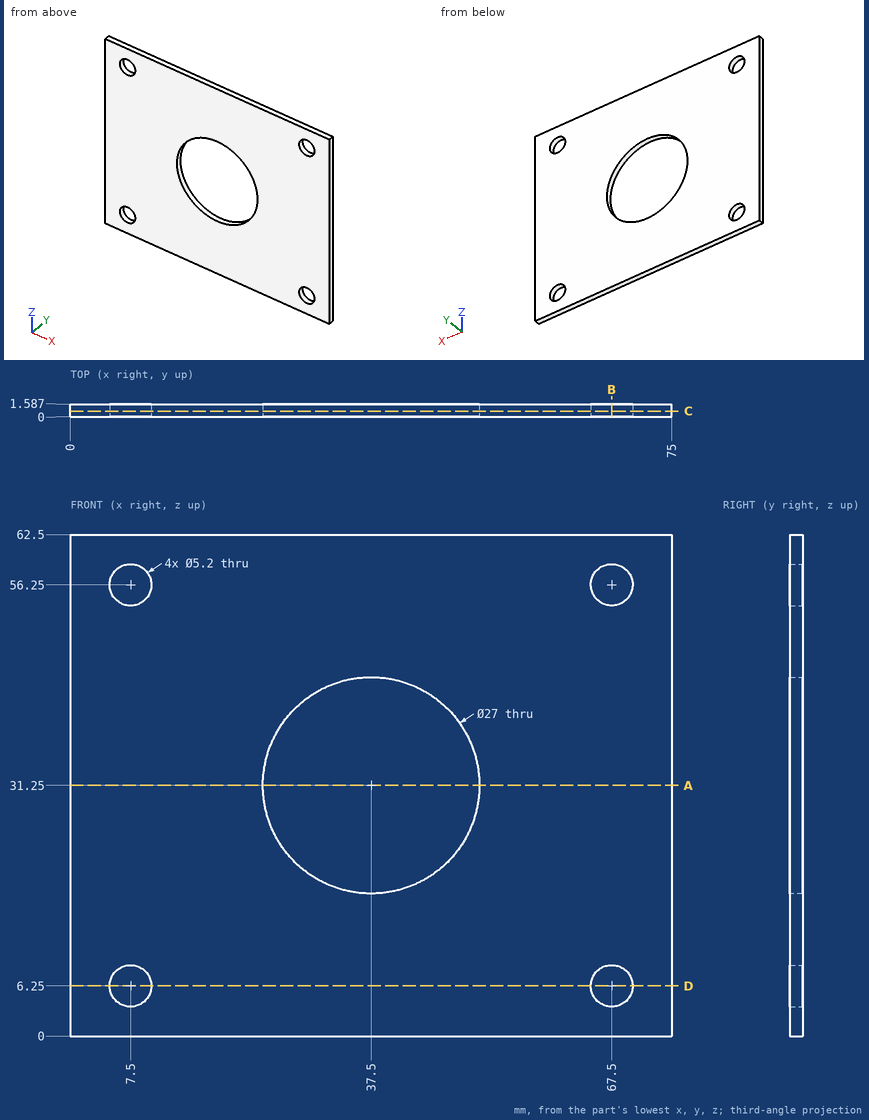
The drawing under review shows one solid part. Ordinate dimensions are in mm from its lowest x, y, z. Round coordinates to 2 decimals unless told otherwise and drop trailing zeros. Order: outer loops, then holes, each group sorted by start corner. A loop starts at its lowest first (then second) coordinate and runs counter-clockwise, first axis right, second up. Notation, with made-up numbers: M 21,30 L 54,30 A28 ccw 54,65 Z; hole C 82,85.5 d8. An arc over 180 degrees is marked long. Answer as CSV lines item,"result". Start each with the question number.
1) Wall thickness on line 1 along Z through (x, y) = (67.5, 1); line 2 along X through (y, z) = (0.6, 6.25); line 3 along Z through (x, y) = (69, 1.45) (1 decimal): over which ranges is each line inside the solid? List them lowest first. Write a range as [from, to].
2) Add section D-D (z = 6.25). Give the boundary of the cut face in (x, y).
3) Add section B-B (x = 67.5). Give the boundary of the cut face in (y, z).
4) Add section C-C (y = 0.7). Give the boundary of the cut face in (x, z).
5) Add section A-A (z = 31.25). Give the boundary of the cut face in (x, y).
Resolved:
1,line 1,"[0, 3.65], [8.85, 53.65], [58.85, 62.5]"
1,line 2,"[0, 4.9], [10.1, 64.9], [70.1, 75]"
1,line 3,"[0, 4.1], [8.4, 54.1], [58.4, 62.5]"
2,outline,"M 0,0 L 4.9,0 L 4.9,1.59 L 0,1.59 Z; M 10.1,0 L 64.9,0 L 64.9,1.59 L 10.1,1.59 Z; M 70.1,0 L 75,0 L 75,1.59 L 70.1,1.59 Z"
3,outline,"M 0,0 L 1.59,0 L 1.59,3.65 L 0,3.65 Z; M 0,8.85 L 1.59,8.85 L 1.59,53.65 L 0,53.65 Z; M 0,58.85 L 1.59,58.85 L 1.59,62.5 L 0,62.5 Z"
4,outline,"M 0,0 L 75,0 L 75,62.5 L 0,62.5 Z; hole C 7.5,6.25 d5.2; hole C 7.5,56.25 d5.2; hole C 37.5,31.25 d27; hole C 67.5,6.25 d5.2; hole C 67.5,56.25 d5.2"
5,outline,"M 0,0 L 24,0 L 24,1.59 L 0,1.59 Z; M 51,0 L 75,0 L 75,1.59 L 51,1.59 Z"
